Can you work these out from the model? Positions are in its coordinate system, mm. Face numbers are marked on the shaded views. A direction names the side the tool comes from. Coordinates: 2 decimals unless noted, no trailing zeros. Order: outer loops, then holes, each group sorted by start corner. A loop starts at its lowest first (then second) coordinate and runs counter-clockwise, first axis right, second up. Notation, with made-up numbers: M 23,86 L 52,86 A29 ccw 52,120 Z; hole C -37.5,65.5 d6. An arc over 180 degrees is marked long. Answer as a JSON object with one key per item and string values.
from build123d import *

# Parameters (mm, degrees)
SKETCH_R             = 11
SKETCH_R_2           = 3
PAD_DEPTH            = 20
POCKET_DEPTH         = 10
SKETCH002_R          = 4
POCKET001_DEPTH      = 8
SKETCH003_R          = 1.5
POCKET002_DEPTH      = 11.001
POCKET002_DEPTH_BACK = -11.001
SKETCH004_W          = 2.5
SKETCH004_H          = 5.6
POCKET003_DEPTH      = 8
SKETCH005_R          = 1.45
POCKET004_DEPTH      = 20.001


with BuildPart() as part:
    # Sketch → Pad (new body)
    with BuildSketch(Plane.XY):
        Circle(SKETCH_R)
        Circle(SKETCH_R_2, mode=Mode.SUBTRACT)
    extrude(amount=PAD_DEPTH)

    # Sketch001 (on Face4 of Pad) → Pocket (cut)
    with BuildSketch(Plane.XY.offset(20)):
        Polygon((-15, -8), (-9, -8), (-9, 9), (9, 9), (9, -9), (-8, -9), (-8, -15), (15, -15), (15, 15), (-15, 15), align=None)
    extrude(amount=-POCKET_DEPTH, mode=Mode.SUBTRACT)

    # Sketch002 (on Face5 of Pocket) → Pocket001 (cut)
    with BuildSketch(Plane.XY.offset(20)):
        Circle(SKETCH002_R)
    extrude(amount=-POCKET001_DEPTH, mode=Mode.SUBTRACT)

    # Sketch003 → Pocket002 (cut, two sides)
    with BuildSketch(Plane.XZ) as pocket002_sk:
        with Locations((0, 5)):
            Circle(SKETCH003_R)
    extrude(amount=-POCKET002_DEPTH, mode=Mode.SUBTRACT)
    extrude(pocket002_sk.sketch, amount=-POCKET002_DEPTH_BACK, mode=Mode.SUBTRACT)

    # Sketch004 (on Face11 of Pocket002) → Pocket003 (cut)
    with BuildSketch(Plane(origin=(0, 0, 0), x_dir=(0, -1, 0), z_dir=(0, 0, -1))):
        with Locations((-5.25, 0)):
            Rectangle(SKETCH004_W, SKETCH004_H)
        with Locations((5.25, 0)):
            Rectangle(SKETCH004_W, SKETCH004_H)
    extrude(amount=-POCKET003_DEPTH, mode=Mode.SUBTRACT)

    # Sketch005 (on Face11 of Pocket003) → Pocket004 (cut, through all)
    with BuildSketch(Plane(origin=(0, 0, 0), x_dir=(1, 0, 0), z_dir=(0, 0, -1))):
        with Locations((-5.5, 5.5)):
            Circle(SKETCH005_R)
        with Locations((-5.5, -5.5)):
            Circle(SKETCH005_R)
        with Locations((5.5, -5.5)):
            Circle(SKETCH005_R)
        with Locations((5.5, 5.5)):
            Circle(SKETCH005_R)
    extrude(amount=-POCKET004_DEPTH, mode=Mode.SUBTRACT)


solid = part.part
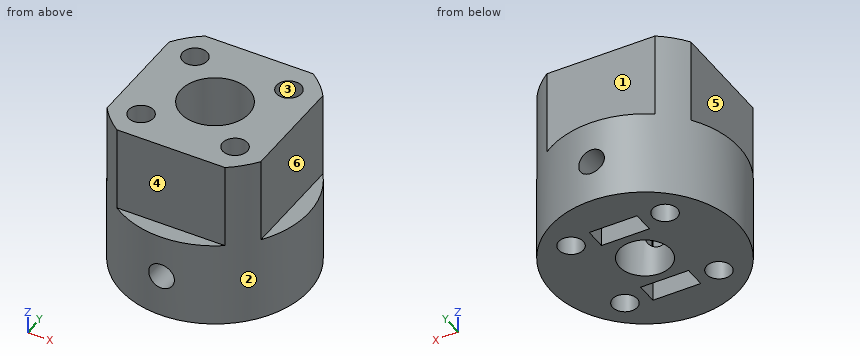
Item 1: I'm going to push flat-ended pins straight in: pin 1 (1.8 mm diameter, centred on x = 0, z = 5, fed in from +Y); pin 2 (2 mm diameter, centred on x = -2.5, z = 2, fed in from +Y); pin 3 (4 mm diameter, centred on x = 0, z = 5, fed in from -Y); pin 4 (1 mm diameter, centred on y = 8, z = 7.5, fed in from -X). Where does each tip first touch, or does it pass through?
Answers follow:
{"pin 1": "passes through", "pin 2": "stops at y = 10.9", "pin 3": "stops at y = -11", "pin 4": "stops at x = -8.05"}
Item 2: Which directions (+Z, -Z, +X, -X, +Y, -Y) give clear straight access to the entire face, cutting with the end or side of a thin tool? Please do the marked faces 4, 5 and 6.
Answers follow:
{"face 4": "+Z, +X, -X, -Y", "face 5": "+Z, -X, +Y, -Y", "face 6": "+Z, +X, +Y, -Y"}
Item 3: If we mould it in two halves opening along Y, with no side actions, what happens to the marked faces 1, 2 and 3? For each: pulls with the +Y half, pulls with the -Y half, needs draft (parallel to the pull), parting line crosses it, or undercut.
Answers follow:
{"face 1": "pulls with the +Y half", "face 2": "parting line crosses it", "face 3": "undercut"}
Item 4: I want a section at B-B, the plane x = 5.5. Write out the boundary of the cut face in (y, z), plus the area to 3 significant figures.
Answers follow:
{"outline": "M -9.53,0 L -6.95,0 L -6.95,20 L -9,20 L -9,10 L -9.53,10 Z; M -4.05,0 L 4.05,0 L 4.05,20 L -4.05,20 Z; M 6.95,0 L 9.53,0 L 9.53,10 L 9,10 L 9,20 L 6.95,20 Z", "area": "255 mm^2"}
Item 5: I want a section at A-A, the plane y = -5.5. Write out the boundary of the cut face in (x, z).
Answers follow:
{"outline": "M -9.53,0 L -6.95,0 L -6.95,20 L -9,20 L -9,10 L -9.53,10 Z; M -4.05,0 L -2.8,0 L -2.8,8 L 2.8,8 L 2.8,0 L 4.05,0 L 4.05,20 L -4.05,20 Z; M 6.95,0 L 9.53,0 L 9.53,10 L 9,10 L 9,20 L 6.95,20 Z"}
Item 6: Please list where these lines run through material, in increasing order: line 1 (Y direction, x = -5.5, z = 10.25); line 2 (Y direction, x = 6.25, z = 9).
Answers follow:
{"line 1": "y = -9 to -6.95, -4.05 to 4.05, 6.95 to 9", "line 2": "y = -9.05 to -6.74, -4.26 to 4.26, 6.74 to 9.05"}
Item 7: I want a section at C-C, the plane z = 15.25. Write out the boundary of the cut face in (x, y), plus the area to 3 significant figures.
Answers follow:
{"outline": "M -9,-6.32 A11 ccw -6.32,-9 L 6.32,-9 A11 ccw 9,-6.32 L 9,6.32 A11 ccw 6.32,9 L -6.32,9 A11 ccw -9,6.32 Z; hole C -5.5,-5.5 d2.9; hole C -5.5,5.5 d2.9; hole C 0,0 d8; hole C 5.5,-5.5 d2.9; hole C 5.5,5.5 d2.9", "area": "235 mm^2"}
Item 8: I want a section at D-D, the plane y = -2.25. Write out the boundary of the cut face in (x, z).
Answers follow:
{"outline": "M -10.77,0 L -1.98,0 L -1.98,12 L -3.31,12 L -3.31,20 L -9,20 L -9,10 L -10.77,10 Z; M 1.98,0 L 10.77,0 L 10.77,10 L 9,10 L 9,20 L 3.31,20 L 3.31,12 L 1.98,12 Z"}
